```python
from build123d import *

# Parameters (mm, degrees)
SKETCH1_W           = 10
SKETCH1_H           = 5.9
BOSS_EXTRUDE1_DEPTH = 5.9
FILLET1_R           = 10
CUT_EXTRUDE1_REACH  = 7.9
SKETCH2_R           = 2.05


with BuildPart() as part:
    # Sketch1 → Boss-Extrude1 (new body)
    with BuildSketch(Plane(origin=(0, 0, 0), x_dir=(1, 0, 0), z_dir=(0, 1, 0))):
        Polygon((-25, 28.925), (-25, -28.925), (0, -28.925), (0, -23.025), (10, -23.025), (10, -28.925), (25, -28.925), (25, 28.925), (10, 28.925), (10, 23.025), (0, 23.025), (0, 28.925), align=None)
        with Locations((5, -25.975)):
            Rectangle(SKETCH1_W, SKETCH1_H)
        with Locations((5, -31.875)):
            Rectangle(SKETCH1_W, SKETCH1_H)
        with Locations((5, 25.975)):
            Rectangle(SKETCH1_W, SKETCH1_H)
        with Locations((5, 31.875)):
            Rectangle(SKETCH1_W, SKETCH1_H)
    extrude(amount=BOSS_EXTRUDE1_DEPTH)

    # Fillet1
    fillet1_edges = [part.edges().sort_by_distance(p)[0] for p in [
        (25, 2.95, -28.925),
        (25, 2.95, 28.925),
        (-25, 2.95, 28.925),
        (-25, 2.95, -28.925),
    ]]
    fillet(fillet1_edges, radius=FILLET1_R)

    # Sketch2 → Cut-Extrude1 (cut, up to next)
    with BuildSketch(Plane(origin=(0, 5.9, 0), x_dir=(1, 0, 0), z_dir=(0, 1, 0)), mode=Mode.PRIVATE) as cut_extrude1_sk1:
        with Locations((0, 28.925)):
            Circle(SKETCH2_R)
    cut_extrude1_tool1 = extrude(cut_extrude1_sk1.sketch, amount=-CUT_EXTRUDE1_REACH, mode=Mode.PRIVATE) & part.part
    add(cut_extrude1_tool1.solids().sort_by_distance((0, 5.9, -28.925))[0], mode=Mode.SUBTRACT)
    # Sketch2 → Cut-Extrude1 (cut, up to next)
    with BuildSketch(Plane(origin=(0, 5.9, 0), x_dir=(1, 0, 0), z_dir=(0, 1, 0)), mode=Mode.PRIVATE) as cut_extrude1_sk2:
        with Locations((10, 28.925)):
            Circle(SKETCH2_R)
    cut_extrude1_tool2 = extrude(cut_extrude1_sk2.sketch, amount=-CUT_EXTRUDE1_REACH, mode=Mode.PRIVATE) & part.part
    add(cut_extrude1_tool2.solids().sort_by_distance((10, 5.9, -28.925))[0], mode=Mode.SUBTRACT)
    # Sketch2 → Cut-Extrude1 (cut, up to next)
    with BuildSketch(Plane(origin=(0, 5.9, 0), x_dir=(1, 0, 0), z_dir=(0, 1, 0)), mode=Mode.PRIVATE) as cut_extrude1_sk3:
        with Locations((0, -28.925)):
            Circle(SKETCH2_R)
    cut_extrude1_tool3 = extrude(cut_extrude1_sk3.sketch, amount=-CUT_EXTRUDE1_REACH, mode=Mode.PRIVATE) & part.part
    add(cut_extrude1_tool3.solids().sort_by_distance((0, 5.9, 28.925))[0], mode=Mode.SUBTRACT)
    # Sketch2 → Cut-Extrude1 (cut, up to next)
    with BuildSketch(Plane(origin=(0, 5.9, 0), x_dir=(1, 0, 0), z_dir=(0, 1, 0)), mode=Mode.PRIVATE) as cut_extrude1_sk4:
        with Locations((10, -28.925)):
            Circle(SKETCH2_R)
    cut_extrude1_tool4 = extrude(cut_extrude1_sk4.sketch, amount=-CUT_EXTRUDE1_REACH, mode=Mode.PRIVATE) & part.part
    add(cut_extrude1_tool4.solids().sort_by_distance((10, 5.9, 28.925))[0], mode=Mode.SUBTRACT)


solid = part.part
```
Read the model definition and answer for the solid it produces. Units are mm, in the model's axes. A direction names the side the tool comes from. Round coordinates to 2 decimals unless told otherwise and drop trailing zeros. Write each loop counter-clockwise with the first axis right and the second up, starting at its lowest first coordinate (ties: lowest second). Pieces come first, ordered by that corner, then holes. Notation, with made-up numbers: M -16,-15 L 16,-15 A21 ccw 16,-8 Z; hole C 58,89.25 d10. An arc over 180 degrees is marked long. One line per item, written item: value.
Q1. Straight lines are drawn through the part: line 1 (Z direction, x = -12.5, y = 0.7) (3 decimals); line 2 (X direction, y = 1.75, z = 21); line 3 (X direction, y = 5.6, z = 26). For each, find the intervals that lie inside material, in ascending order. Write a range as [from, to].
Data:
line 1: [-28.925, 28.925]
line 2: [-24.78, 24.78]
line 3: [-22.07, 22.07]
Q2. Flat-ended cylindrical pins translate along their axes: pin 1 Ø3 at (x, y) = (-13, 5) entering from +Z (3 decimals); pin 2 Ø1 at (y, z) = (3, -22) entering from +X; pin 3 Ø3 at (y, z) = (4, 33.5) entering from +X. Find the tip coordinate at first contact, or state that the pin passes through.
Data:
pin 1: z = 28.925
pin 2: x = 24.66
pin 3: x = 10
Q3. For a pull along X with two mould halves and no side action, classify faces 6 (the cylindrical face through (22.148, 2.991, -25.918)), 7 (the cylindrical face through (8.503, 2.991, -27.524)), 8 (the flat face through (0, 5.9, 0)) as +X half, -X half, draft (parallel to the pull), parting line (faces both ways), or undercut.
Data:
face 6: +X half
face 7: undercut
face 8: draft
Q4. Which of the six approach directions +Z, -Z, +X, -X, +Y, -Y give full straight-line access (tool end or side, diameter ignored) to faces 1 (the flat face through (10, 3, 33)), 2 (the flat face through (0, 3, -33)), 3 (the cylindrical face through (1.4, 2.99, -27.43)), 4 (the flat face through (10, 3, -33)), 5 (the flat face through (0, 3, 33))?
Data:
face 1: +Z, +X, +Y, -Y
face 2: -Z, -X, +Y, -Y
face 3: +Y, -Y
face 4: -Z, +X, +Y, -Y
face 5: +Z, -X, +Y, -Y
Q5. Find section A-A on y = 1.55. Write down the section's boundary in (x, z) (3 decimals).
Data:
outline: M -25,-18.925 A10 ccw -15,-28.925 L -2.05,-28.925 A2.05 cw long 0,-30.975 L 0,-34.825 L 10,-34.825 L 10,-30.975 A2.05 cw long 12.05,-28.925 L 15,-28.925 A10 ccw 25,-18.925 L 25,18.925 A10 ccw 15,28.925 L 12.05,28.925 A2.05 cw long 10,30.975 L 10,34.825 L 0,34.825 L 0,30.975 A2.05 cw long -2.05,28.925 L -15,28.925 A10 ccw -25,18.925 Z
Q6. Find section B-B on x = -1. Write down the section's boundary in (y, z), plus the area to 3 significant figures.
Data:
outline: M 0,-27.14 L 5.9,-27.14 L 5.9,27.14 L 0,27.14 Z
area: 320 mm2
Q7. Find section C-C on x = -17. Write down the section's boundary in (y, z), plus the area to 3 significant figures.
Data:
outline: M 0,-28.72 L 5.9,-28.72 L 5.9,28.72 L 0,28.72 Z
area: 339 mm2
